Design review of the part built by this model. Coordinates are the model's own, in mm. Face numbers are marked on the shaded views. Give positions to 0.01 mm unless a question says otherwise; leave off trailing zeros. Order: outer loops, then holes, each group sorted by start corner. A loop starts at its lowest first (then second) coordinate and runs counter-clockwise, first axis right, second up.
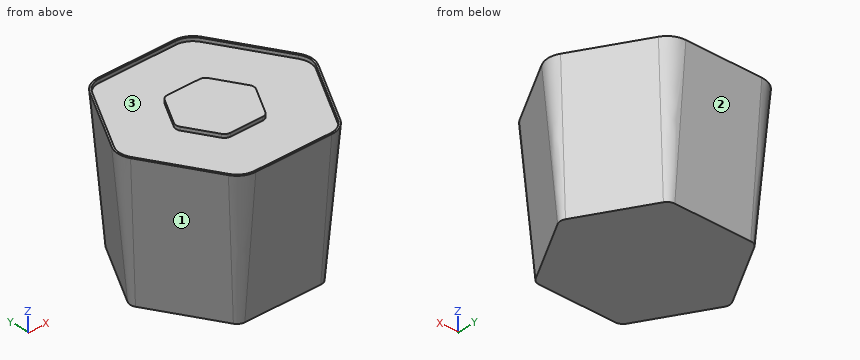
```python
from build123d import *

# Parameters (mm, degrees)
F1_DEPTH = 400
F1_TAPER = 5
F2_DEPTH = 10


with BuildPart() as f1:
    # F0 (on Top) → F1 (new body)
    with BuildSketch(Plane.XY):
        with BuildLine():
            Line((109.696551146, 250), (-109.696551146, 250))
            ThreePointArc((-109.696551146, 250), (-139.696551146, 241.9615242271), (-161.6580753731, 220))
            Line((-161.6580753731, 220), (-271.3546265191, 30))
            ThreePointArc((-271.3546265191, 30), (-279.3931022921, 0), (-271.3546265191, -30))
            Line((-271.3546265191, -30), (-161.6580753731, -220))
            ThreePointArc((-161.6580753731, -220), (-139.696551146, -241.9615242271), (-109.696551146, -250))
            Line((-109.696551146, -250), (109.696551146, -250))
            ThreePointArc((109.696551146, -250), (139.696551146, -241.9615242271), (161.6580753731, -220))
            Line((161.6580753731, -220), (271.3546265191, -30))
            ThreePointArc((271.3546265191, -30), (279.3931022921, 0), (271.3546265191, 30))
            Line((271.3546265191, 30), (161.6580753731, 220))
            ThreePointArc((161.6580753731, 220), (139.696551146, 241.9615242271), (109.696551146, 250))
        make_face()
        with BuildLine():
            ThreePointArc((-109.696551146, -244.9999966036), (-137.1965494478, -237.6313942668), (-157.3279454128, -217.4999983018))
            Line((-157.3279454128, -217.4999983018), (-267.0244965589, -27.4999983018))
            ThreePointArc((-267.0244965589, -27.4999983018), (-274.3930988957, 0), (-267.0244965589, 27.4999983018))
            Line((-267.0244965589, 27.4999983018), (-157.3279454128, 217.4999983018))
            ThreePointArc((-157.3279454128, 217.4999983018), (-137.1965494478, 237.6313942668), (-109.696551146, 244.9999966036))
            Line((-109.696551146, 244.9999966036), (109.696551146, 244.9999966036))
            ThreePointArc((109.696551146, 244.9999966036), (137.1965494478, 237.6313942668), (157.3279454128, 217.4999983018))
            Line((157.3279454128, 217.4999983018), (267.0244965589, 27.4999983018))
            ThreePointArc((267.0244965589, 27.4999983018), (274.3930988957, 0), (267.0244965589, -27.4999983018))
            Line((267.0244965589, -27.4999983018), (157.3279454128, -217.4999983018))
            ThreePointArc((157.3279454128, -217.4999983018), (137.1965494478, -237.6313942668), (109.696551146, -244.9999966036))
            Line((109.696551146, -244.9999966036), (-109.696551146, -244.9999966036))
        make_face(mode=Mode.SUBTRACT)
        with BuildLine():
            Line((-267.0244965589, -27.4999983018), (-157.3279454128, -217.4999983018))
            ThreePointArc((-157.3279454128, -217.4999983018), (-137.1965494478, -237.6313942668), (-109.696551146, -244.9999966036))
            Line((-109.696551146, -244.9999966036), (109.696551146, -244.9999966036))
            ThreePointArc((109.696551146, -244.9999966036), (137.1965494478, -237.6313942668), (157.3279454128, -217.4999983018))
            Line((157.3279454128, -217.4999983018), (267.0244965589, -27.4999983018))
            ThreePointArc((267.0244965589, -27.4999983018), (274.3930988957, 0), (267.0244965589, 27.4999983018))
            Line((267.0244965589, 27.4999983018), (157.3279454128, 217.4999983018))
            ThreePointArc((157.3279454128, 217.4999983018), (137.1965494478, 237.6313942668), (109.696551146, 244.9999966036))
            Line((109.696551146, 244.9999966036), (-109.696551146, 244.9999966036))
            ThreePointArc((-109.696551146, 244.9999966036), (-137.1965494478, 237.6313942668), (-157.3279454128, 217.4999983018))
            Line((-157.3279454128, 217.4999983018), (-267.0244965589, 27.4999983018))
            ThreePointArc((-267.0244965589, 27.4999983018), (-274.3930988957, 0), (-267.0244965589, -27.4999983018))
        make_face()
        with BuildLine():
            ThreePointArc((-63.5085296109, 90), (-56.1880215352, 97.3205080757), (-46.1880215352, 100))
            Line((-46.1880215352, 100), (46.1880215352, 100))
            ThreePointArc((46.1880215352, 100), (56.1880215352, 97.3205080757), (63.5085296109, 90))
            Line((63.5085296109, 90), (109.696551146, 10))
            ThreePointArc((109.696551146, 10), (112.3760430703, 0), (109.696551146, -10))
            Line((109.696551146, -10), (63.5085296109, -90))
            ThreePointArc((63.5085296109, -90), (56.1880215352, -97.3205080757), (46.1880215352, -100))
            Line((46.1880215352, -100), (-46.1880215352, -100))
            ThreePointArc((-46.1880215352, -100), (-56.1880215352, -97.3205080757), (-63.5085296109, -90))
            Line((-63.5085296109, -90), (-109.696551146, -10))
            ThreePointArc((-109.696551146, -10), (-112.3760430703, 0), (-109.696551146, 10))
            Line((-109.696551146, 10), (-63.5085296109, 90))
        make_face(mode=Mode.SUBTRACT)
        with BuildLine():
            Line((46.1880215352, 100), (-46.1880215352, 100))
            ThreePointArc((-46.1880215352, 100), (-56.1880215352, 97.3205080757), (-63.5085296109, 90))
            Line((-63.5085296109, 90), (-109.696551146, 10))
            ThreePointArc((-109.696551146, 10), (-112.3760430703, 0), (-109.696551146, -10))
            Line((-109.696551146, -10), (-63.5085296109, -90))
            ThreePointArc((-63.5085296109, -90), (-56.1880215352, -97.3205080757), (-46.1880215352, -100))
            Line((-46.1880215352, -100), (46.1880215352, -100))
            ThreePointArc((46.1880215352, -100), (56.1880215352, -97.3205080757), (63.5085296109, -90))
            Line((63.5085296109, -90), (109.696551146, -10))
            ThreePointArc((109.696551146, -10), (112.3760430703, 0), (109.696551146, 10))
            Line((109.696551146, 10), (63.5085296109, 90))
            ThreePointArc((63.5085296109, 90), (56.1880215352, 97.3205080757), (46.1880215352, 100))
        make_face()
    extrude(amount=-F1_DEPTH, taper=F1_TAPER)

    # F0 (on Top) → F2 (cut)
    with BuildSketch(Plane.XY):
        with BuildLine():
            Line((-267.0244965589, -27.4999983018), (-157.3279454128, -217.4999983018))
            ThreePointArc((-157.3279454128, -217.4999983018), (-137.1965494478, -237.6313942668), (-109.696551146, -244.9999966036))
            Line((-109.696551146, -244.9999966036), (109.696551146, -244.9999966036))
            ThreePointArc((109.696551146, -244.9999966036), (137.1965494478, -237.6313942668), (157.3279454128, -217.4999983018))
            Line((157.3279454128, -217.4999983018), (267.0244965589, -27.4999983018))
            ThreePointArc((267.0244965589, -27.4999983018), (274.3930988957, 0), (267.0244965589, 27.4999983018))
            Line((267.0244965589, 27.4999983018), (157.3279454128, 217.4999983018))
            ThreePointArc((157.3279454128, 217.4999983018), (137.1965494478, 237.6313942668), (109.696551146, 244.9999966036))
            Line((109.696551146, 244.9999966036), (-109.696551146, 244.9999966036))
            ThreePointArc((-109.696551146, 244.9999966036), (-137.1965494478, 237.6313942668), (-157.3279454128, 217.4999983018))
            Line((-157.3279454128, 217.4999983018), (-267.0244965589, 27.4999983018))
            ThreePointArc((-267.0244965589, 27.4999983018), (-274.3930988957, 0), (-267.0244965589, -27.4999983018))
        make_face()
        with BuildLine():
            ThreePointArc((-63.5085296109, 90), (-56.1880215352, 97.3205080757), (-46.1880215352, 100))
            Line((-46.1880215352, 100), (46.1880215352, 100))
            ThreePointArc((46.1880215352, 100), (56.1880215352, 97.3205080757), (63.5085296109, 90))
            Line((63.5085296109, 90), (109.696551146, 10))
            ThreePointArc((109.696551146, 10), (112.3760430703, 0), (109.696551146, -10))
            Line((109.696551146, -10), (63.5085296109, -90))
            ThreePointArc((63.5085296109, -90), (56.1880215352, -97.3205080757), (46.1880215352, -100))
            Line((46.1880215352, -100), (-46.1880215352, -100))
            ThreePointArc((-46.1880215352, -100), (-56.1880215352, -97.3205080757), (-63.5085296109, -90))
            Line((-63.5085296109, -90), (-109.696551146, -10))
            ThreePointArc((-109.696551146, -10), (-112.3760430703, 0), (-109.696551146, 10))
            Line((-109.696551146, 10), (-63.5085296109, 90))
        make_face(mode=Mode.SUBTRACT)
    extrude(amount=-F2_DEPTH, mode=Mode.SUBTRACT)


solid = f1.part
```
1. For line 1 along Y through (x, z) = (-55, -62.5); line 2 along Z through (x, y) = (81.5, 126.5); line 3 along Y through (x, z) = (251.5, -105.5), list the stretches that pass through material, from the lowest coordinate up.
Recorded:
line 1: y = -244.53 to 244.53
line 2: z = -400 to -10
line 3: y = -45.93 to 45.93
2. Take a section at D-D (x = -199.5). State the section outline as (y, z) points, then the cut area to 3 significant figures.
Recorded:
outline: (-154.46, 0) - (-84.46, -400) - (84.46, -400) - (154.46, 0) - (144.46, 0) - (144.46, -10) - (-144.46, -10) - (-144.46, 0) - close
area: 92,700 mm2
3. Draft analysis for pull direction X (two halves, no side actions). For the marked faces 1, 2 and 3, state which applies: pulls with the +X half, pulls with the -X half, needs draft (parallel to the pull), parting line crosses it, or undercut.
Recorded:
face 1: pulls with the -X half
face 2: needs draft
face 3: undercut
4. Take a section at C-C (z = -84). State the section outline as (x, y) points, then the cut area to 3 significant figures.
Recorded:
outline: (-264.99, -26.33) - (-155.29, -216.33) arc R52.65 ccw to (-109.7, -242.65) - (109.7, -242.65) arc R52.65 ccw to (155.29, -216.33) - (264.99, -26.33) arc R52.65 ccw to (264.99, 26.33) - (155.29, 216.33) arc R52.65 ccw to (109.7, 242.65) - (-109.7, 242.65) arc R52.65 ccw to (-155.29, 216.33) - (-264.99, 26.33) arc R52.65 ccw to start
area: 203,000 mm2
5. Take a section at B-B (y = 148.5). State the section outline as (x, z) points, then the cut area to 3 significant figures.
Recorded:
outline: (-202.94, 0) - (-162.53, -400) - (162.53, -400) - (202.94, 0) - (197.17, 0) - (197.17, -10) - (-197.17, -10) - (-197.17, 0) - close
area: 142,000 mm2
6. For pin 1 (12 mm diameter, centred on x = 73.5, z = -225, fed in from -Y); pin 2 (6 mm diameter, centred on y = 59.5, z = -302.5, fed in from +X); pin 3 (10 mm diameter, centred on x = 73, y = 164.5, fed in from +Z), all flat-tipped, find the tip position at first contact; note any pin that passes through.
Recorded:
pin 1: stops at y = -230.84
pin 2: stops at x = 225.52
pin 3: stops at z = -10
7. Take a section at A-A (x = 33). State the section outline as (y, z) points, then the cut area to 3 significant figures.
Recorded:
outline: (-250, 0) - (-215, -400) - (215, -400) - (250, 0) - (245, 0) - (245, -10) - (100, -10) - (100, 0) - (-100, 0) - (-100, -10) - (-245, -10) - (-245, 0) - close
area: 183,000 mm2
